Geometry: final body of the model. Coordinates: model frame, mm. Face numbers are marked on the shaded views. Round coordinates to 2 decimals unless told otherwise and drop trailing zeros. Write each loop counter-clockwise with the first axis right and the second up, starting at its lowest first coordinate (ties: lowest second). Pieces come first, ordered by that corner, then holes. Notation, with made-up numbers: M -30,56 L 26,56 A22 cw 26,85 Z; hole C 43.25,13.5 d6. An arc over 180 degrees is marked long. Answer as CSV lines item,"result". Start each with the question number.
Q1. Section query C-C on y = 9.75. Output: boundary loops of the cut face in (x, z).
Q2. Ray query, probe 1 along X at (y, z) = (23.75, -165.1); probe 2 along X at (y, z) = (6.25, 128.5); probe 3 along X at (y, z) = (2.25, -74). Return the intervals inside material, ascending.
Q3. Mould query, pull axis Z, two halves, no side actions, for the marked faces 1 and 2. Classes: pulls with the +Z half, pulls with the -Z half, needs draft (parallel to the pull), parting line crosses it, or undercut.
Q4. Section query D-D on z = 171. Output: boundary loops of the cut face in (x, y).
Q5. Section query A-A on z = -39. Output: boundary loops of the cut face in (x, y), and give its area (3 significant figures).
Q6. Section query B-B on x = 224. Output: boundary loops of the cut face in (y, z), and give its area (3 significant figures).
Q7. First-contact query: pin 1 (1 mm diameter, centred on x = 27.5, y = 3, fed in from -Z); pin 2 (3 mm diameter, centred on x = -150, z = 47, fed in from -Y); pin 3 (4 mm diameter, centred on x = -167.56, z = -165.1, fed in from +Y). Flat tips, straight axial feed; report the tip coordinate or a pass-through.
```python
from build123d import *

# Parameters (mm, degrees)
BOSS_EXTRUDE1_DEPTH = 25.4
FILLET1_R           = 20.32
SHELL1_T            = -2.54
SKETCH2_R           = 2.54
CUT_EXTRUDE1_DEPTH  = 347.409815103


with BuildPart() as part:
    # Sketch1 → Boss-Extrude1 (new body)
    with BuildSketch(Plane(origin=(0, 0, 0), x_dir=(1, 0, 0), z_dir=(0, 1, 0))):
        Polygon((-279.4, 203.2), (-279.4, -203.2), (279.4, -203.2), (279.4, 203.2), (152.4, 203.2), (152.4, 12.7), (-152.4, 12.7), (-152.4, 203.2), align=None)
    extrude(amount=BOSS_EXTRUDE1_DEPTH)

    # Fillet1
    fillet1_edges = [part.edges().sort_by_distance(p)[0] for p in [
        (279.4, 12.7, -203.2),
        (-279.4, 12.7, -203.2),
        (-152.4, 12.7, -203.2),
        (152.4, 12.7, -203.2),
    ]]
    fillet(fillet1_edges, radius=FILLET1_R)

    # Shell1
    shell1_openings = [part.faces().sort_by_distance(p)[0] for p in [
        (0, 0, 37.577423361),
    ]]
    offset(amount=SHELL1_T, openings=shell1_openings, kind=Kind.INTERSECTION)

    # Sketch2 → Cut-Extrude1 (cut, through all)
    with BuildSketch(Plane(origin=(0, 25.4, 0), x_dir=(1, 0, 0), z_dir=(0, 1, 0))):
        with Locations(Location((-177.72, 165.1, 0), (0, 0, 270))):
            Circle(SKETCH2_R)
        with Locations(Location((-167.56, 165.1, 0), (0, 0, 270))):
            Circle(SKETCH2_R)
        with Locations(Location((167.56, 165.1, 0), (0, 0, 270))):
            Circle(SKETCH2_R)
        with Locations(Location((177.72, 165.1, 0), (0, 0, 270))):
            Circle(SKETCH2_R)
    extrude(amount=-CUT_EXTRUDE1_DEPTH, mode=Mode.SUBTRACT)


solid = part.part
```
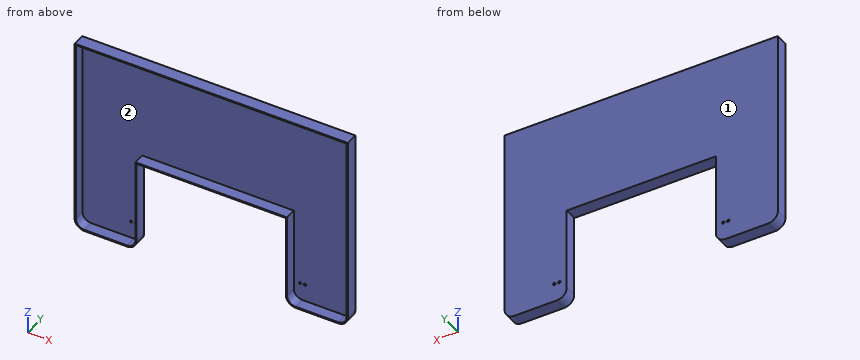
Entries:
1,outline,"M -279.4,-182.88 A20.32 ccw -259.08,-203.2 L -172.72,-203.2 A20.32 ccw -152.4,-182.88 L -152.4,-12.7 L 152.4,-12.7 L 152.4,-182.88 A20.32 ccw 172.72,-203.2 L 259.08,-203.2 A20.32 ccw 279.4,-182.88 L 279.4,203.2 L -279.4,203.2 Z; hole M -276.86,-182.88 A17.78 ccw -259.08,-200.66 L -172.72,-200.66 A17.78 ccw -154.94,-182.88 L -154.94,-10.16 L 154.94,-10.16 L 154.94,-182.88 A17.78 ccw 172.72,-200.66 L 259.08,-200.66 A17.78 ccw 276.86,-182.88 L 276.86,200.66 L -276.86,200.66 Z"
2,probe 1,"x = -279.4 to -180.26, -175.18 to -170.1, -165.02 to -152.4, 152.4 to 165.02, 170.1 to 175.18, 180.26 to 279.4"
2,probe 2,"x = -279.4 to -276.86, 276.86 to 279.4"
2,probe 3,"x = -279.4 to -276.86, -154.94 to -152.4, 152.4 to 154.94, 276.86 to 279.4"
3,face 1,"needs draft"
3,face 2,"undercut"
4,outline,"M -279.4,0 L -276.86,0 L -276.86,22.86 L 276.86,22.86 L 276.86,0 L 279.4,0 L 279.4,25.4 L -279.4,25.4 Z"
5,outline,"M -279.4,0 L -276.86,0 L -276.86,22.86 L -154.94,22.86 L -154.94,0 L -152.4,0 L -152.4,25.4 L -279.4,25.4 Z; M 152.4,0 L 154.94,0 L 154.94,22.86 L 276.86,22.86 L 276.86,0 L 279.4,0 L 279.4,25.4 L 152.4,25.4 Z"
5,area,"877 mm^2"
6,outline,"M 0,-203.2 L 25.4,-203.2 L 25.4,203.2 L 0,203.2 L 0,200.66 L 22.86,200.66 L 22.86,-200.66 L 0,-200.66 Z"
6,area,"1,150 mm^2"
7,pin 1,"stops at z = -12.7"
7,pin 2,"stops at y = 22.86"
7,pin 3,"passes through"
